from build123d import *

# Parameters (mm, degrees)
SCHIZZO1_W                   = 148
SCHIZZO1_H                   = 42
ESTRUSIONE_ESTRUSIONE1_DEPTH = 2
SCHIZZO2_W                   = 148
SCHIZZO2_H                   = 42
SCHIZZO2_W_2                 = 144
SCHIZZO2_H_2                 = 38
ESTRUSIONE_ESTRUSIONE2_DEPTH = 6
SCHIZZO3_W                   = 2
SCHIZZO3_H                   = 10
ESTRUSIONE_ESTRUSIONE3_DEPTH = 6
ESTRUSIONE_ESTRUSIONE3_TAPER = 3


with BuildPart() as part:
    # Schizzo1 → Estrusione-Estrusione1 (new body)
    with BuildSketch(Plane.XY):
        Rectangle(SCHIZZO1_W, SCHIZZO1_H)
    extrude(amount=ESTRUSIONE_ESTRUSIONE1_DEPTH)

    # Schizzo2 → Estrusione-Estrusione2 (add)
    with BuildSketch(Plane.XY.offset(2)):
        Rectangle(SCHIZZO2_W, SCHIZZO2_H)
        Rectangle(SCHIZZO2_W_2, SCHIZZO2_H_2, mode=Mode.SUBTRACT)
    extrude(amount=ESTRUSIONE_ESTRUSIONE2_DEPTH)

    # Schizzo3 → Estrusione-Estrusione3 (add)
    with BuildSketch(Plane.XY.offset(8)):
        with Locations((-73, 0.515392861)):
            Rectangle(SCHIZZO3_W, SCHIZZO3_H)
    estrusione_estrusione3 = extrude(amount=ESTRUSIONE_ESTRUSIONE3_DEPTH, taper=ESTRUSIONE_ESTRUSIONE3_TAPER)

    # Specchia1: Estrusione-Estrusione3 across plane
    add(estrusione_estrusione3.mirror(Plane(origin=(0, 0, 0), x_dir=(0, 0, 1), z_dir=(1, 0, 0))))


solid = part.part
Model file for the job. Use its own axes, mm. A direction names the side the tool comes from. Coordinates: 2 decimals unless noted, no trailing zeros. Order: outer loops, then holes, each group sorted by start corner. A loop starts at its lowest first (then second) coordinate and runs counter-clockwise, first axis right, second up. Notation, with made-up numbers: (-7.5, 31.5) -> (22.5, 31.5) arc R15 ccw to (22.5, 39.5) -> close; hole circle Ø7 at (-22.5, 9). An arc over 180 degrees is marked (long way). Return JSON: item names as keys, results as strings. Group by question number.
Item 1: Flat gauge pins, fed straight in: P1, Ø7.5, axis at x = 6.5, y = 16, coming from the +Z side; P2, Ø1.5, axis at x = -53, y = 0, coming from the +Z side; P3, Ø4, axis at y = 5.5, z = 10.5, coming from the +X side. Where does each tip first touch, or does it go through?
Item 2: Saw through at A-A on z = 12.5. Write the cut outline in (x, y).
Item 3: Saw through at C-C on y = 9. Write the cut outline in (x, z), then the cut area to 3 significant figures.
Item 4: Wall check: line 1 along Y through (x, z) = (48.5, 3); line 2 along X through (y, z) = (-4, 4.75); line 3 along Z through (x, y) = (65, 4.5). Give the ranges that are in metal, low to high. Write a range as [from, to].
Item 5: Tool access for faces 1 (the flat face through (-72.155, 0.585, 10.958)), 2 (the flat face through (74, 0, 4)), 3 (the flat face through (-72, 0, 5)): list every direction of +Z, -Z, +X, -X, +Y, -Y with a clear straight run to the whole face (end or side of a thin tool).
Item 6: Saw through at D-D on x = 60.5. Write the cut outline in (y, z).
Item 7: Saw through at B-B on z = 4.25. Write the cut outline in (x, y), then the cut area to 3 significant figures.
Item 8: Pull direction X, two halves, no side cores. Call faces 4 (the flat face through (-1, 0, 2)), 5 (the flat face through (72.155, 0.585, 10.958)), 6 (the flat face through (73.845, 0.445, 10.958)), 7 (the flat face through (-1, -21, 4)): pulls with the +X half, pulls with the -X half, needs draft (parallel to the pull), parting line crosses it, or undercut.
Values found:
{
 "1": {"P1": "stops at z = 8", "P2": "stops at z = 2", "P3": "stops at x = 73.97"},
 "2": {"outline": "(-73.76, -4.25) -> (-72.24, -4.25) -> (-72.24, 5.28) -> (-73.76, 5.28) -> close; (72.24, -4.25) -> (73.76, -4.25) -> (73.76, 5.28) -> (72.24, 5.28) -> close"},
 "3": {"outline": "(-74, 0) -> (74, 0) -> (74, 8) -> (72, 8) -> (72, 2) -> (-72, 2) -> (-72, 8) -> (-74, 8) -> close", "area": "320 mm2"},
 "4": {"line 1": "y = [-21, -19], [19, 21]", "line 2": "x = [-74, -72], [72, 74]", "line 3": "z = [0, 2]"},
 "5": {"face 1": "+Z, +Y, -Y", "face 2": "+Z, -Z, +X, +Y, -Y", "face 3": "+Z"},
 "6": {"outline": "(-21, 0) -> (21, 0) -> (21, 8) -> (19, 8) -> (19, 2) -> (-19, 2) -> (-19, 8) -> (-21, 8) -> close"},
 "7": {"outline": "(-74, -21) -> (74, -21) -> (74, 21) -> (-74, 21) -> close; hole (-72, -19) -> (72, -19) -> (72, 19) -> (-72, 19) -> close", "area": "744 mm2"},
 "8": {"face 4": "undercut", "face 5": "undercut", "face 6": "pulls with the +X half", "face 7": "needs draft"}
}
